Part model, mm, in its own coordinate system. A direction names the side the tool comes from. Coordinates: 2 decimals unless noted, no trailing zeros. Order: outer loops, then holes, each group sorted by start corner. A loop starts at its lowest first (then second) coordinate and runs counter-clockwise, first axis right, second up.
from build123d import *

# Parameters (mm, degrees)
F0_W      = 420
F0_H      = 420
F1_DEPTH  = 105
F2_T      = -6
F3_W      = 6
F3_H      = 408
F4_DEPTH  = 18
F5_W      = 6
F5_H      = 408
F6_DEPTH  = 18
F7_W      = 6
F7_H      = 18
F8_DEPTH  = 372
F9_W      = 6
F9_H      = 18
F10_DEPTH = 372
F11_W     = 408
F11_H     = 408
F11_W_2   = 400
F11_H_2   = 400
F12_DEPTH = 10
F14_DEPTH = 25.4
F15_W     = 400
F15_H     = 400
F16_DEPTH = 10


with BuildPart() as f1:
    # F0 (on Front) → F1 (new body, symmetric)
    with BuildSketch(Plane.XZ):
        Rectangle(F0_W, F0_H)
    extrude(amount=F1_DEPTH, both=True)

    # F2
    f2_openings = [f1.faces().sort_by_distance(p)[0] for p in [
        (0, -105, 0),
    ]]
    offset(amount=F2_T, openings=f2_openings)

    # F3 (on face) → F4 (join)
    with BuildSketch(Plane.YZ.offset(-204)):
        with Locations((-92, 0)):
            Rectangle(F3_W, F3_H)
    extrude(amount=F4_DEPTH)

    # F5 (on face) → F6 (join)
    with BuildSketch(Plane(origin=(204, 0, 0), x_dir=(0, -1, 0), z_dir=(-1, 0, 0))):
        with Locations((92, 0)):
            Rectangle(F5_W, F5_H)
    extrude(amount=F6_DEPTH)

    # F7 (on face) → F8 (join, through all)
    with BuildSketch(Plane.YZ.offset(-186)):
        with Locations((-92, 195)):
            Rectangle(F7_W, F7_H)
    extrude(amount=F8_DEPTH)

    # F9 (on face) → F10 (join, through all)
    with BuildSketch(Plane.YZ.offset(-186)):
        with Locations((-92, -195)):
            Rectangle(F9_W, F9_H)
    extrude(amount=F10_DEPTH)

    # F11 (on face) → F12 (join)
    with BuildSketch(Plane.XZ.offset(95)):
        Rectangle(F11_W, F11_H)
        Rectangle(F11_W_2, F11_H_2, mode=Mode.SUBTRACT)
    extrude(amount=F12_DEPTH)

    # F13: F1 across face


with BuildPart() as f1_1:
    add(f1.part)
    add(f1.part.mirror(Plane(origin=(0, 105, 0), x_dir=(1, 0, 0), z_dir=(0, 1, 0))))

    # F14 (cut): a face of the model
    f14_faces = [f1_1.faces().sort_by_distance(p)[0] for p in [
        (0, 111, 0),
    ]]
    extrude(f14_faces, amount=-F14_DEPTH, mode=Mode.SUBTRACT)

    # F15 (on face) → F16 (join)
    with BuildSketch(Plane(origin=(0, 305, 0), x_dir=(-1, 0, 0), z_dir=(0, 1, 0))):
        Rectangle(F15_W, F15_H)
    extrude(amount=F16_DEPTH)


solid = f1_1.part
Q1. Wall check: line 1 along Z through (x, y) = (-137.5, 145.5); line 2 along Y through (x, z) = (-142, 55). Give the ranges that are in metal, low to high.
Results list:
line 1: z = -210 to -204, 204 to 210
line 2: y = 305 to 315
Q2. Mould opens along Y. For faces 1 (the face through (210, 108, -3)), 2 (the face through (3, 305, 3)), 3 (the face through (195, 299, -16)) say: pulls with the +Y half, pulls with the -Y half, needs draft (parallel to the pull), parting line crosses it, or undercut.
Results list:
face 1: needs draft
face 2: pulls with the -Y half
face 3: undercut
Q3. Which spindle directions (+Z, -Z, +X, -X, +Y, -Y) get a long thin tool onto all of the face, cutting with end or side? Do faces 4 (the face through (-3, 108, -204)), 5 (the face through (-3, 108, -210)), 6 (the face through (192, -95, -16)). Say none if no direction does.
Results list:
face 4: none
face 5: -Z, +X, -X, +Y, -Y
face 6: -Y
Q4. Pin check, flat tip, straight feed: pin 1 Ø8 at (x, z) = (-41.5, 13) entering from -Y. Stop position of the tip, or through.
Results list:
pin 1: stops at y = 305
Q5. Cut at C-C on x = 15. Write the cut outline in (y, z), and give its area (3 significant figures).
Results list:
outline: (-105, -210) - (315, -210) - (315, 210) - (-105, 210) - (-105, 200) - (-95, 200) - (-95, 186) - (-89, 186) - (-89, 204) - (299, 204) - (299, 186) - (305, 186) - (305, -186) - (299, -186) - (299, -204) - (-89, -204) - (-89, -186) - (-95, -186) - (-95, -200) - (-105, -200) - close
area: 9,630 mm2
Q6. Cut at A-A on y = -50. Write the cut outline in (x, z), and give its area (3 significant figures).
Results list:
outline: (-210, -210) - (210, -210) - (210, 210) - (-210, 210) - close; hole (-204, -204) - (204, -204) - (204, 204) - (-204, 204) - close
area: 9,940 mm2
Q7. Cut at B-B on z = 160. Write the cut outline in (x, y), and give its area (3 significant figures).
Results list:
outline: (-210, -105) - (-200, -105) - (-200, -95) - (-186, -95) - (-186, -89) - (-204, -89) - (-204, 299) - (-186, 299) - (-186, 305) - (186, 305) - (186, 299) - (204, 299) - (204, -89) - (186, -89) - (186, -95) - (200, -95) - (200, -105) - (210, -105) - (210, 315) - (-210, 315) - close
area: 9,630 mm2
